```python
from build123d import *

# Parameters (mm, degrees)
F0_W     = 133.7834484875
F0_H     = 72.8662703186
F1_DEPTH = 76.2
F2_W     = 115.2523923665
F2_H     = 59.2436287552
F3_DEPTH = 72.8672703186
F4_R     = 10.8422221272
F5_DEPTH = 133.7844484875
F6_W     = 66.7222347111
F6_H     = 33.3499126136
F7_DEPTH = 76.201


with BuildPart() as f1:
    # F0 (on Front) → F1 (new body)
    with BuildSketch(Plane.XZ):
        with Locations((-32.7633004636, -15.3782842681)):
            Rectangle(F0_W, F0_H)
    extrude(amount=-F1_DEPTH)

    # F2 (on face) → F3 (cut, through all)
    with BuildSketch(Plane.XY.offset(21.0548508912)):
        with Locations((-33.0736329779, 39.0397785231)):
            Rectangle(F2_W, F2_H)
    extrude(amount=-F3_DEPTH, mode=Mode.SUBTRACT)

    # F4 (on face) → F5 (cut, through all)
    with BuildSketch(Plane.YZ.offset(34.1284237802)):
        with Locations((42.7399463952, -14.2118474469)):
            Circle(F4_R)
    extrude(amount=-F5_DEPTH, mode=Mode.SUBTRACT)

    # F6 (on face) → F7 (cut, through all)
    with BuildSketch(Plane.XZ):
        with Locations((-22.6808311418, 16.6749563068)):
            Rectangle(F6_W, F6_H)
    extrude(amount=-F7_DEPTH, mode=Mode.SUBTRACT)


solid = f1.part
```
Build history of the part. All positions in model axes, mm. A direction names the side the tool comes from. Give positions to 0.01 mm unless a question says otherwise; leave off trailing zeros. Loops run counter-clockwise (first coordinate to the right, second up) from the corner with the lowest first, then second, coordinate; pieces in that order, holes last. Notation, with made-up numbers: (60.25, 56.5) -> (99.25, 56.5) arc R9 cw to (99.25, 66.5) -> close; hole circle Ø7 at (17.5, 71.25). An arc over 180 degrees is marked (long way). One line per question, with ' | ' between items. Start each with the question number.
1) Cut at B-B (x = -9). Give the cut face in (y, z).
2) Pin check, flat tip, straight feed: pin 1 (4.5 mm diameter, centred on x = -9.5, y = 3.5, fed in from +Z). Stop position of the tip, or through.
3) 3-axis set-ups, long thin cutter, end or side, ignore diameter. For faces 1 (the flat face through (-99.655, 37.6, -24)), 2 (the flat face through (24.553, 32, -7)), 3 (the flat face through (10.68, 5, 10)): which of +Z, -Z, +X, -X, +Y, -Y reach the whole face in a straight line?
4) Cut at A-A (y = 12). Give the cut face in (x, z), plus the area to 3 significant figures.
5) Cut at C-C (z = 6). Give the cut face in (x, y), plus the area to 3 significant figures.
6) Two-plate mould, pull along Y, no slides. Class faces 4 (the flat face through (-23, 5, 0)), 5 (the flat face through (-90.7, 32, -7)), 6 (the flat face through (-34, 0, -23)): released by +Y, released by -Y, zero draft, split by the parting line, or undercut.
7) Probe L1, parallel to X at y = 48, z = 2; L2, parallel to Y at x = -89, z = -26. List the from-to ranges inside material, lowest first.
8) Cut at D-D (z = -34). Give the cut face in (x, y), plus the area to 3 significant figures.
Return value:
1) outline: (0, -51.81) -> (9.42, -51.81) -> (9.42, 0) -> (0, 0) -> close; (68.66, -51.81) -> (76.2, -51.81) -> (76.2, 0) -> (68.66, 0) -> close
2) pin 1: z = 0
3) face 1: +Z, -Z, -X, +Y, -Y | face 2: +Z, -Z | face 3: +Z, +Y, -Y
4) outline: (-99.66, -51.81) -> (-90.7, -51.81) -> (-90.7, 21.05) -> (-99.66, 21.05) -> close; (24.55, -51.81) -> (34.13, -51.81) -> (34.13, 21.05) -> (24.55, 21.05) -> close | area: 1,350 mm^2
5) outline: (-99.66, 0) -> (-56.04, 0) -> (-56.04, 9.42) -> (-90.7, 9.42) -> (-90.7, 68.66) -> (-56.04, 68.66) -> (-56.04, 76.2) -> (-99.66, 76.2) -> close; (10.68, 0) -> (34.13, 0) -> (34.13, 76.2) -> (10.68, 76.2) -> (10.68, 68.66) -> (24.55, 68.66) -> (24.55, 9.42) -> (10.68, 9.42) -> close | area: 2,230 mm^2
6) face 4: zero draft | face 5: undercut | face 6: released by -Y
7) L1: -99.66 to -90.7, 24.55 to 34.13 | L2: 0 to 9.42, 68.66 to 76.2
8) outline: (-99.66, 0) -> (34.13, 0) -> (34.13, 76.2) -> (-99.66, 76.2) -> close; hole (-90.7, 9.42) -> (24.55, 9.42) -> (24.55, 68.66) -> (-90.7, 68.66) -> close | area: 3,370 mm^2
